Can you work these out from the model? Positions are in its coordinate system, mm. Face numbers are marked on the shaded views. Round coordinates to 2 decimals unless told otherwise and drop trailing zeros. Loops run counter-clockwise (first coordinate to the right, second up) from the corner with the lowest first, then second, coordinate; pieces in that order, holes last. Notation, with made-up numbers: (78.25, 83.5) - (118.25, 83.5) arc R22 ccw to (118.25, 93.5) - close; hole circle Ø7 at (-7, 86.25). An arc over 180 degrees is marked (long way). Answer as CSV lines item,"result".
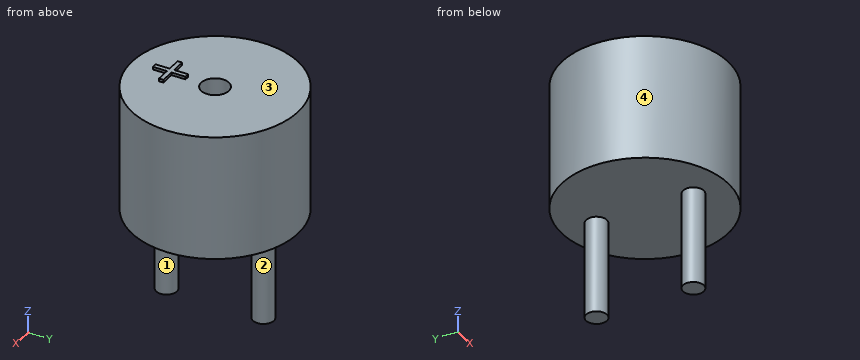
Autodesk Inventor part; units mm, degrees
ref_plane "YZ Plane" through (0, 0, 0) normal (1, 0, 0) x (0, 1, 0)
ref_plane "XZ Plane" through (0, 0, 0) normal (0, 1, 0) x (-1, 0, 0)
ref_plane "XY Plane" through (0, 0, 0) normal (0, 0, 1) x (1, 0, 0)
sketch "Sketch1" plane through (0, 0, 0) normal (0, 0, 1) x (1, 0, 0)
  circle A0 centre (0, 0) radius 6
  dimension "d0" = 12
extrude "Extrusion1" add sketch "Sketch1" along normal blind 9
sketch "Sketch2" plane through (0, 0, 9) normal (0, 0, 1) x (1, 0, 0)
  circle A0 centre (0, 0) radius 1
  line L0 (-2.0016, -1.6454) -> (2.0016, -1.6454) construction
  line L1 (2.0016, -1.6454) -> (2.0016, -4.7864) construction
  line L2 (2.0016, -4.7864) -> (-2.0016, -4.7864) construction
  line L3 (-2.0016, -4.7864) -> (-2.0016, -1.6454) construction
  line L4 (1.1852, -3.3776) -> (0.169, -3.3776)
  line L5 (0.169, -3.3776) -> (0.169, -4.3938)
  line L6 (0.169, -4.3938) -> (-0.1665, -4.3938)
  line L7 (-0.1665, -4.3938) -> (-0.1665, -3.3776)
  line L8 (-0.1665, -3.3776) -> (-1.1827, -3.3776)
  line L9 (-1.1827, -3.3776) -> (-1.1827, -3.0543)
  line L10 (-1.1827, -3.0543) -> (-0.1665, -3.0543)
  line L11 (-0.1665, -3.0543) -> (-0.1665, -2.0381)
  line L12 (-0.1665, -2.0381) -> (0.169, -2.0381)
  line L13 (0.169, -2.0381) -> (0.169, -3.0543)
  line L14 (0.169, -3.0543) -> (1.1852, -3.0543)
  line L15 (1.1852, -3.0543) -> (1.1852, -3.3776)
  point P0 (0, -1.6454)
  dimension "d3" = 2
extrude "Extrusion2" cut sketch "Sketch2" against normal blind 5 contours A0
extrude "Extrusion3" add sketch "Sketch2" along normal blind 0.2 contours L4 L5 L6 L7 L8 L9 L10 L11 L12 L13 L14 L15
sketch "Sketch3" plane through (0, 0, 0) normal (0, 0, -1) x (-1, 0, 0)
  circle A0 centre (0, 3.5) radius 0.75
  circle A1 centre (0, -3.5) radius 0.75
  line L0 (0, 3.5) -> (0, -3.5) construction
  point P0 (0, 0)
  point P1 (0, 0)
  dimension "d8" = 1.5
  dimension "d9" = 7
extrude "Extrusion4" add sketch "Sketch3" along normal blind 7
properties part number "Buzzer" material "PBT Plastic"
Q1. Imagine slicing it at C-C (z = 6.5). Write out the boundary of the cut face in (x, y), then the cut area to 3 significant figures.
Checks:
outline,"circle Ø12 at (0, 0); hole circle Ø2 at (0, 0)"
area,"110 mm²"
Q2. We'd pull the mould along Y, two halves only. Please class the marked faces 1, 2, 3 and 4: pulls with the +Y half, pulls with the -Y half, needs draft (parallel to the pull), parting line crosses it, or undercut.
Checks:
face 1,"undercut"
face 2,"undercut"
face 3,"needs draft"
face 4,"parting line crosses it"
Q3. Imagine slicing it at B-B (z = -2.5). Write out the boundary of the cut face in (x, y), then the cut area to 3 significant figures.
Checks:
outline,"circle Ø1.5 at (0, -3.5); circle Ø1.5 at (0, 3.5)"
area,"3.53 mm²"
Q4. Imagine slicing it at D-D (x = -5). Write out the boundary of the cut face in (y, z), then the cut area to 3 significant figures.
Checks:
outline,"(-3.32, 0) - (3.32, 0) - (3.32, 9) - (-3.32, 9) - close"
area,"59.7 mm²"
Q5. Imagine slicing it at A-A (y = 0). Write out the boundary of the cut face in (x, z).
Checks:
outline,"(-6, 0) - (6, 0) - (6, 9) - (1, 9) - (1, 4) - (-1, 4) - (-1, 9) - (-6, 9) - close"
Q6. If I drill on line 1 along Y through (x, z) = (0, 6.85); line 2 along Z through (x, y) = (3, 3.75); line 3 along Y through (x, z) = (-1, 1.25), over which ranges is the centre line in solid material (lowest first)? Write a range as [from, to].
Checks:
line 1,"[-6, -1], [1, 6]"
line 2,"[0, 9]"
line 3,"[-5.92, 5.92]"
Q7. I'm going to push flat-ended pins straight in: pin 1 Ø6 at (y, z) = (2, -3.5) entering from -X; pin 2 Ø1.6 at (x, y) = (0, 0) entering from -Z; pin 3 Ø3 at (x, y) = (0.5, 4.5) entering from +Z; pin 4 Ø1.5 at (y, z) = (0.5, -4) entering from +X. Where does each tip first touch, or does it pass through?
Checks:
pin 1,"x = -0.75"
pin 2,"z = 0"
pin 3,"z = 9"
pin 4,"through"
